Work out the finished part from the listing and answer in its coordinate system (mm). Face numbers are marked on the shaded views. A direction names the side the tool comes from. Coordinates: 2 decimals unless noted, no trailing zeros. Write each loop counter-clockwise with the first axis right and the second up, starting at its lowest first coordinate (ties: lowest second). Pieces come first, ordered by that corner, then holes. Notation, with made-up numbers: (41.5, 8) - (83.5, 8) arc R25 cw to (83.5, 25) - close; hole circle Ø4 at (35, 42). An arc over 180 degrees is marked (long way). Use a Markdown table: item, result. Add a question column.
(1) The part is cut by section D-D, the plane y = 18.5. Give the vertices of the cut face in (x, z), then the cut area to 3 significant figures.
(2) For a pull along Z with two mould halves and no side action, classify the marked faces 5, 6 and 7 as released by +Z, released by -Z, zero draft, split by the parting line, or undercut.
(3) The part is cut by section C-C, the plane z = 28.5. Give the vertices of the cut face in (x, y), then the cut area to 3 significant figures.
(4) A tool of negligible diameter and unlimited length cuts with its end or side. For the marked faces 1, 2, 3 and 4, from which of +Z, -Z, +X, -X, +Y, -Y can it reach the whole face along a straight path? Write none if from no direction.
(5) The part is cut by section A-A, the plane y = 6.5. Give the vertices of the cut face in (x, z).
(6) Given pin 1 Ø19 at (x, y) = (1.5, 7.5) entering from -Z; pin 2 Ø1.5 at (x, y) = (-12, -15) entering from -Z; pin 3 Ø24 at (y, z) = (-2.5, 9) entering from +X, each flat-ended and moving along its own axis, determine where each tip first touches the part or whether it passes through.
(7) Find the intervals of material crossed by line 1 (Y direction, x = 0, z = 1.9); line 2 (Z direction, x = -11.5, y = 15.5); line 3 (X direction, y = 15, z = 29.15), in increasing order. Write a range as from..to.
(8) The part is cut by section B-B, the plane x = 0. Give the vertices of the cut face in (y, z).
from build123d import *

# Parameters (mm, degrees)
F1_DEPTH = 30
F2_R     = 20
F2_W     = 24
F2_H     = 30
F3_DEPTH = 30
F4_W     = 15
F4_H     = 22
F5_DEPTH = 25.4


with BuildPart() as f1:
    # F0 (on Top) → F1 (new body)
    with BuildSketch(Plane.XY):
        with BuildLine():
            Line((7.5, 15), (12, 15))
            ThreePointArc((12, 15), (0, 27), (-12, 15))
            Line((-12, 15), (-7.5, 15))
            ThreePointArc((-7.5, 15), (0, 22.5), (7.5, 15))
        make_face()
        with BuildLine():
            ThreePointArc((-12, 15), (0, 3), (12, 15))
            Line((12, 15), (7.5, 15))
            ThreePointArc((7.5, 15), (0, 7.5), (-7.5, 15))
            Line((-7.5, 15), (-12, 15))
        make_face()
        with BuildLine():
            Line((12, -15), (12, 15))
            ThreePointArc((12, 15), (0, 3), (-12, 15))
            Line((-12, 15), (-12, -15))
            Line((-12, -15), (12, -15))
        make_face()
    extrude(amount=F1_DEPTH)

    # F2 (on face) → F3 (join)
    with BuildSketch(Plane.XZ.offset(15)):
        with Locations((0, 15)):
            Circle(F2_R)
        with Locations((0, 15)):
            Rectangle(F2_W, F2_H, mode=Mode.SUBTRACT)
        with Locations((0, 15)):
            Rectangle(F2_W, F2_H)
    extrude(amount=F3_DEPTH)

    # F4 (on face) → F5 (cut)
    with BuildSketch(Plane(origin=(-12, 0, 0), x_dir=(0, -1, 0), z_dir=(-1, 0, 0))):
        with Locations((-22.5, 15)):
            Rectangle(F4_W, F4_H)
        with Locations((-7.5, 15)):
            Rectangle(F4_W, F4_H)
    extrude(amount=-F5_DEPTH, mode=Mode.SUBTRACT)


solid = f1.part
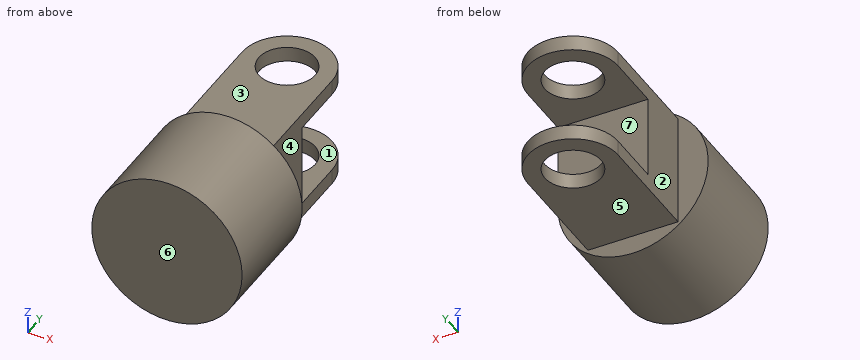
Model answer:
| question | item | result |
|---|---|---|
| 1 | outline | (-11.48, 0) - (-6.63, 0) - (-6.63, 4) - (-11.48, 4) - close; (-11.48, 26) - (-6.63, 26) - (-6.63, 30) - (-11.48, 30) - close; (6.63, 0) - (11.48, 0) - (11.48, 4) - (6.63, 4) - close; (6.63, 26) - (11.48, 26) - (11.48, 30) - (6.63, 30) - close |
| 1 | area | 77.5 mm^2 |
| 2 | face 5 | released by -Z |
| 2 | face 6 | zero draft |
| 2 | face 7 | undercut |
| 3 | outline | (-14.76, -45) - (14.76, -45) - (14.76, -15) - (12, -15) - (12, 15) arc R12 ccw to (-12, 15) - (-12, -15) - (-14.76, -15) - close; hole circle Ø15 at (0, 15) |
| 3 | area | 1,650 mm^2 |
| 4 | face 1 | +X, -X, +Y |
| 4 | face 2 | +Z, -Z, -X, +Y |
| 4 | face 3 | +Z, +X, -X, +Y |
| 4 | face 4 | +Z, -Z, +X, +Y |
| 5 | outline | (-12, 0) - (12, 0) - (12, 4) - (-12, 4) - close; (-12, 26) - (12, 26) - (12, 30) - (-12, 30) - close |
| 6 | pin 1 | z = 0 |
| 6 | pin 2 | z = -1.54 |
| 6 | pin 3 | x = 12 |
| 7 | line 1 | -45..7.5, 22.5..27 |
| 7 | line 2 | 0..4, 26..30 |
| 7 | line 3 | -12..-7.5, 7.5..12 |
| 8 | outline | (-45, -5) - (-15, -5) - (-15, 0) - (7.5, 0) - (7.5, 4) - (0, 4) - (0, 26) - (7.5, 26) - (7.5, 30) - (-15, 30) - (-15, 35) - (-45, 35) - close; (22.5, 0) - (27, 0) - (27, 4) - (22.5, 4) - close; (22.5, 26) - (27, 26) - (27, 30) - (22.5, 30) - close |
